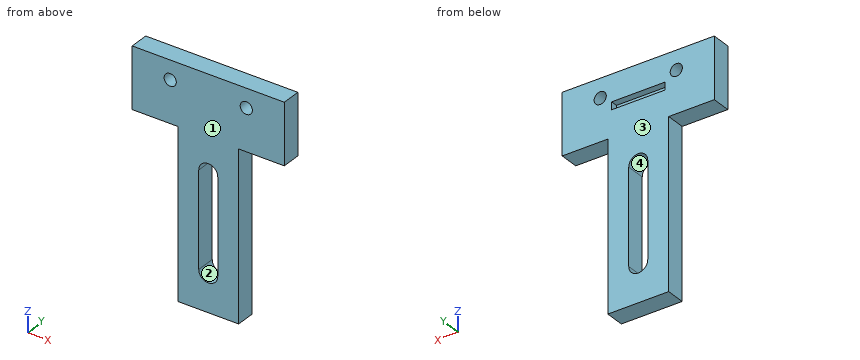
```python
from build123d import *

# Parameters (mm, degrees)
SKETCH_2_R          = 1.6
EXTRUDE_2_DEPTH     = 5
CUT_EXTRUDE_1_DEPTH = 56.009090158
SKETCH_6_W          = 14
SKETCH_6_H          = 2
CUT_EXTRUDE_2_DEPTH = 1.8


with BuildPart() as part:
    # 草图2 → 凸台-拉伸2 (new body)
    with BuildSketch(Plane(origin=(0, 0, 0), x_dir=(1, 0, 0), z_dir=(0, 1, 0))):
        Polygon((-20, 16), (-8, 16), (-8, 60), (8, 60), (8, 16), (20, 16), (20, 0), (-20, 0), align=None)
        with Locations(Location((-10, 5, 0), (0, 0, 270))):
            Circle(SKETCH_2_R, mode=Mode.SUBTRACT)
        with Locations(Location((10, 5, 0), (0, 0, 270))):
            Circle(SKETCH_2_R, mode=Mode.SUBTRACT)
    extrude(amount=-EXTRUDE_2_DEPTH)

    # 草图5 → 切除-拉伸1 (cut, through all)
    with BuildSketch(Plane(origin=(0, -5, -9), x_dir=(1, 0, 0), z_dir=(0, 1, 0))):
        with BuildLine():
            Line((2.5, 41), (2.5, 16))
            ThreePointArc((2.5, 16), (0, 13.5), (-2.5, 16))
            Line((-2.5, 16), (-2.5, 41))
            ThreePointArc((-2.5, 41), (0, 43.5), (2.5, 41))
        make_face()
    extrude(amount=CUT_EXTRUDE_1_DEPTH, mode=Mode.SUBTRACT)

    # 草图6 → 切除-拉伸2 (cut)
    with BuildSketch(Plane(origin=(0, 0, 0), x_dir=(1, 0, 0), z_dir=(0, 1, 0))):
        with Locations((0, 8)):
            Rectangle(SKETCH_6_W, SKETCH_6_H)
    extrude(amount=-CUT_EXTRUDE_2_DEPTH, mode=Mode.SUBTRACT)


solid = part.part
```
Check sheet for the modelled part. Datum: model origin and axes. Units: mm. Face numbers are marked on the shaded views. A direction names the side the tool comes from. Give positions to 0.01 mm unless a question says otherwise; leave off trailing zeros. Write each loop counter-clockwise with the first axis right and the second up, starting at its lowest first coordinate (ties: lowest second). Pieces come first, ordered by that corner, then holes. Notation, with made-up numbers: (47.25, 73.5) - (86.25, 73.5) arc R23 cw to (86.25, 96.5) - close; hole circle Ø3 at (10.25, 55.5). An arc over 180 degrees is marked (long way). Answer as a JSON object with one key per item and string values. Group by question number.
1) Sectioned sample at C-C (y = -1.05). Record the cut outline in (x, z).
2) Access from +Z, -Z, +X, -X, +Y, -Y to the whole of each face (thin tool, end or side, straight path). Record for the marked faces 1 and 2.
3) Sectioned sample at D-D (z = -49). Record the cut outline in (x, y), then the cut area to 3 significant figures.
4) Depth check by flat-ended pin: P1, Ø12, axis at x = -16, z = -23.5, coming from the +Y side; P2, Ø1.5, axis at x = 15.5, y = -2.5, coming from the -Z side; P3, Ø0.6, axis at x = 2.5, z = -8, coming from the +Y side; P4, Ø2.5, axis at y = -1.5, z = -32, coming from the +X side. Enter the tip coordinate at first touch or a pass-through.
5) Sectioned sample at B-B (z = -5). Record the cut outline in (x, y).
6) Release check for a two-part mould opening along X. For the marked faces 3 and 4 record: pulls with the +X half, pulls with the -X half, needs draft (parallel to the pull), parting line crosses it, or undercut.
7) Thickness scan on probe 1 along X at (y, z) = (-2.4, -5); probe 2 along X at (y, z) = (-4.15, -42.5); probe 3 along Z at (x, y) = (-5.5, -1.2). Record the ranges inside material, lowest first. Write a range as from..to.
8) Sectioned sample at A-A (x = 0). Record the cut outline in (y, z).
Geometry results:
{
 "1": {"outline": "(-20, -16) - (-8, -16) - (-8, -60) - (8, -60) - (8, -16) - (20, -16) - (20, 0) - (-20, 0) - close; hole circle Ø3.2 at (-10, -5); hole (-7, -9) - (7, -9) - (7, -7) - (-7, -7) - close; hole (-2.5, -50) arc R2.5 ccw to (2.5, -50) - (2.5, -25) arc R2.5 ccw to (-2.5, -25) - close; hole circle Ø3.2 at (10, -5)"},
 "2": {"face 1": "+Z, -Z, +X, -X, -Y", "face 2": "+Y, -Y"},
 "3": {"outline": "(-8, -5) - (-2.5, -5) - (-2.5, 0) - (-8, 0) - close; (2.5, -5) - (8, -5) - (8, 0) - (2.5, 0) - close", "area": "55.0 mm^2"},
 "4": {"P1": "passes through", "P2": "stops at z = -16", "P3": "stops at y = -1.8", "P4": "stops at x = 8"},
 "5": {"outline": "(-20, -5) - (-11.6, -5) - (-11.6, 0) - (-20, 0) - close; (-8.4, -5) - (8.4, -5) - (8.4, 0) - (-8.4, 0) - close; (11.6, -5) - (20, -5) - (20, 0) - (11.6, 0) - close"},
 "6": {"face 3": "needs draft", "face 4": "undercut"},
 "7": {"probe 1": "x = -20..-11.6, -8.4..8.4, 11.6..20", "probe 2": "x = -8..-2.5, 2.5..8", "probe 3": "z = -60..-9, -7..0"},
 "8": {"outline": "(-5, -60) - (0, -60) - (0, -52.5) - (-5, -52.5) - close; (-5, -22.5) - (0, -22.5) - (0, -9) - (-1.8, -9) - (-1.8, -7) - (0, -7) - (0, 0) - (-5, 0) - close"}
}
